Verification items for the finished model (mm, model axes). Give positions to 0.01 mm unless a question says otherwise; leave off trailing zeros. Loops run counter-clockwise (first coordinate to the right, second up) from the corner with the lowest first, then second, coordinate; pieces in that order, holes last. Notation, with made-up numbers: (-31.5, 30) - (8.5, 30) arc R15 cw to (8.5, 48) - close; hole circle Ø7 at (-20.75, 55). An arc over 180 degrees is marked (long way). Use one line per item in the form item = value.
```python
from build123d import *

# Parameters (mm, degrees)
SKETCH1_R           = 17.5
SKETCH1_R_2         = 3.4
SKETCH1_R_3         = 2.731026391
BOSS_EXTRUDE1_DEPTH = 6
FILLET1_R           = 8
CUT_EXTRUDE5_DEPTH  = 10
CUT_EXTRUDE6_DEPTH  = 10
FILLET2_R           = 8
CHAMFER1_SIZE       = 5.15
CUT_EXTRUDE7_DEPTH  = 10
FILLET3_R           = 2


with BuildPart() as part:
    # Sketch1 → Boss-Extrude1 (new body)
    with BuildSketch(Plane(origin=(0, 0, 0), x_dir=(1, 0, 0), z_dir=(0, 1, 0))):
        Polygon((-175, 275), (-225, -275), (225, -275), (175, 275), align=None)
        with Locations(Location((0, 215, 0), (0, 0, 270))):
            Circle(SKETCH1_R, mode=Mode.SUBTRACT)
        with Locations(Location((-145.777131586, 243, 0), (0, 0, 270))):
            Circle(SKETCH1_R_2, mode=Mode.SUBTRACT)
        with Locations(Location((145.777131586, 243, 0), (0, 0, 90))):
            Circle(SKETCH1_R_2, mode=Mode.SUBTRACT)
        with Locations(Location((-189.958949768, -243, 0), (0, 0, 270))):
            Circle(SKETCH1_R_2, mode=Mode.SUBTRACT)
        with Locations(Location((189.958949768, -243, 0), (0, 0, 90))):
            Circle(SKETCH1_R_2, mode=Mode.SUBTRACT)
        with Locations(Location((-167.868040677, 0, 0), (0, 0, 270))):
            Circle(SKETCH1_R_2, mode=Mode.SUBTRACT)
        with Locations(Location((167.868040677, 0, 0), (0, 0, 90))):
            Circle(SKETCH1_R_2, mode=Mode.SUBTRACT)
        with Locations(Location((0, 115, 0), (0, 0, 270))):
            Circle(SKETCH1_R_3, mode=Mode.SUBTRACT)
    extrude(amount=-BOSS_EXTRUDE1_DEPTH)

    # Fillet1
    fillet1_edges = [part.edges().sort_by_distance(p)[0] for p in [
        (175, -3, -275),
        (225, -3, 275),
        (-225, -3, 275),
        (-175, -3, -275),
    ]]
    fillet(fillet1_edges, radius=FILLET1_R)

    # Sketch6 → Cut-Extrude5 (cut)
    with BuildSketch(Plane(origin=(0, 0, 0), x_dir=(1, 0, 0), z_dir=(0, 1, 0))):
        Polygon((-204.631966366, -95.133074099), (-182.722315824, 145.873081867), (-194.245635018, 159.701064899), (-218.459949399, -106.656393293), align=None)
    cut_extrude5 = extrude(amount=-CUT_EXTRUDE5_DEPTH, mode=Mode.SUBTRACT)

    # Sketch7 → Cut-Extrude6 (cut)
    with BuildSketch(Plane(origin=(0, 0, 0), x_dir=(1, 0, 0), z_dir=(0, 1, 0))):
        Polygon((-31.320564901, -271.594250629), (31.320564901, -271.594250629), (45, -279.893229805), (-45, -279.893229805), align=None)
    extrude(amount=-CUT_EXTRUDE6_DEPTH, mode=Mode.SUBTRACT)

    # Mirror2: Cut-Extrude5 across plane
    add(cut_extrude5.mirror(Plane(origin=(0, 0, 0), x_dir=(0, 0, 1), z_dir=(1, 0, 0))), mode=Mode.SUBTRACT)

    # Fillet2
    fillet2_edges = [part.edges().sort_by_distance(p)[0] for p in [
        (36.934355042, -3, 275),
        (-36.934355042, -3, 275),
        (-31.320564901, -3, 271.594250629),
        (31.320564901, -3, 271.594250629),
        (204.631966366, -3, 95.133074099),
        (182.722315824, -3, -145.873081867),
        (-182.722315824, -3, -145.873081867),
        (-204.631966366, -3, 95.133074099),
    ]]
    fillet(fillet2_edges, radius=FILLET2_R)

    # Chamfer1
    chamfer1_edges = [part.edges().sort_by_distance(p)[0] for p in [
        (-145.777131586, 0, -246.4),
        (145.777131586, 0, -239.6),
        (-189.958949768, 0, 239.6),
        (189.958949768, 0, 246.4),
        (-167.868040677, 0, -3.4),
        (167.868040677, 0, 3.4),
    ]]
    chamfer(chamfer1_edges, length=CHAMFER1_SIZE)

    # Sketch11 → Cut-Extrude7 (cut)
    with BuildSketch(Plane(origin=(0, 0, 0), x_dir=(1, 0, 0), z_dir=(0, 1, 0))):
        with BuildLine():
            Line((-179.910507926, 220.984412813), (-169.951575861, 220.079055353))
            ThreePointArc((-169.951575861, 220.079055353), (-165.334252813, 214.538267695), (-170.875040471, 209.920944647))
            Line((-170.875040471, 209.920944647), (-180.833972536, 210.826302107))
            Line((-180.833972536, 210.826302107), (-179.910507926, 220.984412813))
        make_face()
        with BuildLine():
            Line((-219.001417017, -209.015587187), (-209.042484952, -209.920944647))
            ThreePointArc((-209.042484952, -209.920944647), (-204.425161904, -215.461732305), (-209.965949562, -220.079055353))
            Line((-209.965949562, -220.079055353), (-219.924881627, -219.173697893))
            Line((-219.924881627, -219.173697893), (-219.001417017, -209.015587187))
        make_face()
        with BuildLine():
            Line((219.001417017, -209.015587187), (219.924881627, -219.173697893))
            Line((219.924881627, -219.173697893), (209.965949562, -220.079055353))
            ThreePointArc((209.965949562, -220.079055353), (204.425161904, -215.461732305), (209.042484952, -209.920944647))
            Line((209.042484952, -209.920944647), (219.001417017, -209.015587187))
        make_face()
        with BuildLine():
            Line((179.910507926, 220.984412813), (180.833972536, 210.826302107))
            Line((180.833972536, 210.826302107), (170.875040471, 209.920944647))
            ThreePointArc((170.875040471, 209.920944647), (165.334252813, 214.538267695), (169.951575861, 220.079055353))
            Line((169.951575861, 220.079055353), (179.910507926, 220.984412813))
        make_face()
    extrude(amount=-CUT_EXTRUDE7_DEPTH, mode=Mode.SUBTRACT)

    # Fillet3
    fillet3_edges = [part.edges().sort_by_distance(p)[0] for p in [
        (-180.833972536, -3, -210.826302107),
        (-179.910507926, -3, -220.984412813),
        (-219.924881627, -3, 219.173697893),
        (-219.001417017, -3, 209.015587187),
        (179.910507926, -3, -220.984412813),
        (180.833972536, -3, -210.826302107),
        (219.001417017, -3, 209.015587187),
        (219.924881627, -3, 219.173697893),
    ]]
    fillet(fillet3_edges, radius=FILLET3_R)


solid = part.part
```
1. Section check B-B, the plane z = -84. Record the cut outline in (x, y).
Result set:
outline = (-188.35, -6) - (188.35, -6) - (188.35, 0) - (-188.35, 0) - close
2. Section check A-A, the plane y = -1.5. State how many separate pieces and enclosed holes the cut face has, then the cut area to 3 significant figures.
Result set:
separate_pieces = 1
enclosed_holes = 8
area = 215,000 mm²
3. Scan lines: probe 1 along X at (y, z) = (-5.75, -243); probe 2 along X at (y, z) = (-5.7, 0); probe 3 along X at (y, z) = (-1.9, -215). Record each from-to range of solid material in increasing order.
Result set:
probe_1 = -177.91 to -149.18, -142.38 to 142.38, 149.18 to 177.91
probe_2 = -195.98 to -171.27, -164.47 to 164.47, 171.27 to 195.98
probe_3 = -165.31 to -17.5, 17.5 to 165.31
4. Section check C-C, the plane z = 120.5. Record the cut outline in (x, y), then the cut area to 3 significant figures.
Result set:
outline = (-210.95, -6) - (210.95, -6) - (210.95, 0) - (-210.95, 0) - close
area = 2,530 mm²
5. Depth check by flat-ended pin: pin 1 Ø3 at (y, z) = (-3.5, 40.5) entering from +X; pin 2 Ø3 at (x, y) = (-7, -4) entering from +Z; pin 3 Ø9 at (x, z) = (189.96, 243) entering from +Y; pin 4 Ø8.5 at (x, z) = (0, -115) entering from -Y. Enter the tip coordinate at first touch or a pass-through.
Result set:
pin_1 = 199.8
pin_2 = 271.59
pin_3 = -4.05
pin_4 = -6
6. Draft check along Z on faces 1 (the conical face through (171.43, -4.9, 0.79)), 2 (the flat face through (-3, 0, -4)), 3 (the cylindrical face through (0.769, -2.958, -232.483)). Enter one of: released by +Z, released by -Z, zero draft, split by the parting line, or undercut.
Result set:
face_1 = undercut
face_2 = zero draft
face_3 = undercut
